Autodesk Inventor part; units mm, degrees
ref_plane "YZ Plane" through (0, 0, 0) normal (1, 0, 0) x (0, 1, 0)
ref_plane "XZ Plane" through (0, 0, 0) normal (0, 1, 0) x (-1, 0, 0)
ref_plane "XY Plane" through (0, 0, 0) normal (0, 0, 1) x (1, 0, 0)
sketch "Sketch1" plane through (0, 0, 0) normal (0, 1, 0) x (-1, 0, 0)
  line L0 (-4.6, -6) -> (-4.6, 0)
  line L1 (0, -6) -> (-4.6, -6)
  line L2 (0, 0) -> (0, -6)
  line L3 (0, 0) -> (-4.6, 0)
  line L4 (37.7, -0.1) -> (-42.3, -0.1)
  line L5 (-42.3, -0.1) -> (-42.3, -5.9)
  line L6 (-42.3, -5.9) -> (37.7, -5.9)
  line L7 (37.7, -5.9) -> (37.7, -0.1)
  line L8 (-2.3, -6) -> (-2.3, 0) construction
  dimension "d0" = 0.1
  dimension "d1" = 0.1
  dimension "d2" = 80
extrude "Extrusion1" add sketch "Sketch1" along normal blind 2.9 contours L6 L5 L4 L0 | L0 L4 L2 L6 | L2 L4 L7 L6
sketch "Sketch3" plane through (0, 0, 0) normal (0, -1, 0) x (1, 0, 0)
  line L0 (42.3, -5.9) -> (-37.7, -5.9)
  line L1 (-37.7, -0.1) -> (42.3, -0.1)
  line L2 (39.3, -5.9) -> (36.3, -5.9)
  line L3 (36.3, -5.9) -> (36.3, -0.1)
  line L4 (36.3, -0.1) -> (39.3, -0.1)
  line L5 (39.3, -0.1) -> (39.3, -5.9)
  line L6 (39.3, -4.5) -> (36.3, -4.5)
  line L7 (36.3, -4.5) -> (36.3, -1.5)
  line L8 (36.3, -1.5) -> (39.3, -1.5)
  line L9 (39.3, -1.5) -> (39.3, -4.5)
  line L10 (39.3, -3) -> (36.3, -3) construction
  line L11 (42.3, -0.1) -> (42.3, -5.9)
  point P0 (0, 0)
  dimension "d5" = 3
  dimension "d6" = 3
extrude "Extrusion2" cut sketch "Sketch3" against normal through all contours L6 L3 L8 L5
extrude "Extrusion3" cut sketch "Sketch3" against normal blind 1.5 contours L0 L3 L6 L5 | L5 L8 L3 L1
pattern_linear "Rectangular Pattern1" count 5 spacing 6 along (-1, 0, 0) of "Extrusion3", "Extrusion2"
ref_plane "Work Plane1" through (2.3, 0, -0.1) normal (1, 0, 0) x (0, 0, -1)
mirror "Mirror1" about plane through (2.3, 0, -0.1) normal (1, 0, 0) of "Extrusion3", "Extrusion2", "Rectangular Pattern1"
equation "\"d0\" = slack"
equation "\"d1\" = slack"
equation "\"slack\" = 0.1"
properties part number "Slider"
For this review, take the finished solid that the model builds, in its own axes (mm). A direction names the side the tool comes from. Coordinates: 2 decimals unless noted, no trailing zeros. Loops run counter-clockwise (first coordinate to the right, second up) from the corner with the lowest first, then second, coordinate; pieces in that order, holes last. Notation, with made-up numbers: (28.25, 58) - (55.25, 58) arc R24 ccw to (55.25, 70) - close; hole circle Ø3 at (5.25, 14). An arc over 180 degrees is marked (long way). Use one line per item in the form item = value. Start each with the question number.
1) Take a section at A-A (x = 13.5). State the section outline as (y, z) points, plus the area to 3 significant figures.
2) Take a section at B-B (z = -3.85). State how many separate pieces and enclosed holes the cut face has, plus the area to 3 significant figures.
3) For pin 1 (0.7 mm diameter, centred on x = -8.5, z = -5.5, fed in from -Y), flat-tipped, find the tip position at first contact; note if it passes through.
4) To check wall thickness, follow probe 1 along Z at (x, y) = (-14.5, 2); probe 2 along Y at (x, z) = (38.5, -4.85). State the ranges of each line that lie inside material, in increasing order. Write a range as from..to.
5) For faces 1 (the face through (26, 2, -1.5)), 2 (the face through (14, 1.5, -1)), 3 (the face through (-22.7, 1, -3)), list the 3-axis set-ups (+Z, -Z, +X, -X, +Y, -Y) from which the entire face can be reached by the end or side of a thin tool; tool diameter is ignored.
6) Draft analysis for pull direction Z (two halves, no side actions). For faces 4 (the face through (36.3, 1, -3)), 5 (the face through (-15, 1.5, -1)), state which applies: released by +Z, released by -Z, zero draft, split by the parting line, or undercut.
From the geometry:
q1.outline = (1.5, -5.9) - (2.9, -5.9) - (2.9, -4.5) - (1.5, -4.5) - close; (1.5, -1.5) - (2.9, -1.5) - (2.9, -0.1) - (1.5, -0.1) - close
q1.area = 3.92 mm2
q2.separate_pieces = 11
q2.enclosed_holes = 0
q2.area = 145 mm2
q3.pin_1 = 1.5
q4.probe_1 = -5.9..-4.5, -1.5..-0.1
q4.probe_2 = 1.5..2.9
q5.face_1 = +Y, -Y
q5.face_2 = +Z, -Z, -Y
q5.face_3 = -Y
q6.face_4 = undercut
q6.face_5 = zero draft
